from build123d import *

# Parameters (mm, degrees)
F0_W     = 127
F0_H     = 254
F1_DEPTH = 101.6
F3_DEPTH = 101.601


with BuildPart() as f1:
    # F0 (on Front) → F1 (new body)
    with BuildSketch(Plane.XZ):
        with Locations((-70.0115717482, 66.6608795685)):
            Rectangle(F0_W, F0_H)
    extrude(amount=F1_DEPTH)

    # F2 (on face) → F3 (cut, through all)
    with BuildSketch(Plane.XZ.offset(101.6)):
        with BuildLine():
            ThreePointArc((-133.5115717482, 89.8414792443), (-90.6735324782, 69.9836491161), (-61.4159074664, 107.0433631539))
            ThreePointArc((-61.4159074664, 107.0433631539), (-90.6735324782, 144.1030771918), (-133.5115717482, 124.2452470636))
            Line((-133.5115717482, 124.2452470636), (-133.5115717482, 89.8414792443))
        make_face()
    extrude(amount=-F3_DEPTH, mode=Mode.SUBTRACT)


solid = f1.part
Build history of the part. All positions in model axes, mm. Round coordinates to 2 decimals unless told otherwise and drop trailing zeros. Loops run counter-clockwise (first coordinate to the right, second up) from the corner with the lowest first, then second, coordinate; pieces in that order, holes last. Notation, with made-up numbers: (46, 45) -> (72, 45) arc R15 ccw to (72, 50) -> close; hole circle Ø3 at (46.5, -25). An arc over 180 degrees is marked (long way). Answer in a Markdown table with one row per item.
Item 1: Drill centre lines: L1, parallel to Z at x = -97.5, y = -71; L2, parallel to Z at x = -65.5, y = -63; L3, parallel to X at y = -79, z = 83. Where is each one in solid material? Low to high. Write a range as [from, to].
Answers below:
| item | result |
|---|---|
| L1 | z = [-60.34, 69], [145.09, 193.66] |
| L2 | z = [-60.34, 89.88], [124.21, 193.66] |
| L3 | x = [-133.51, -129.07], [-69.96, -6.51] |
Item 2: Saw through at C-C (z = 135). Write the cut outline in (x, y), and give its area (3 significant figures).
Answers below:
| item | result |
|---|---|
| outline | (-133.51, -101.6) -> (-125.4, -101.6) -> (-125.4, 0) -> (-133.51, 0) -> close; (-73.63, -101.6) -> (-6.51, -101.6) -> (-6.51, 0) -> (-73.63, 0) -> close |
| area | 7,640 mm² |
Item 3: Saw through at D-D (z = 99.5). Write the cut outline in (x, y), and give its area (3 significant figures).
Answers below:
| item | result |
|---|---|
| outline | (-62.17, -101.6) -> (-6.51, -101.6) -> (-6.51, 0) -> (-62.17, 0) -> close |
| area | 5,650 mm² |
Item 4: Saw through at A-A (x = -87). Write the cut outline in (y, z), and give its area (3 significant figures).
Answers below:
| item | result |
|---|---|
| outline | (-101.6, -60.34) -> (0, -60.34) -> (0, 71.06) -> (-101.6, 71.06) -> close; (-101.6, 143.03) -> (0, 143.03) -> (0, 193.66) -> (-101.6, 193.66) -> close |
| area | 18,500 mm² |
Item 5: Saw through at B-B (y = -48). Write the cut outline in (x, z), and give its area (3 significant figures).
Answers below:
| item | result |
|---|---|
| outline | (-133.51, -60.34) -> (-6.51, -60.34) -> (-6.51, 193.66) -> (-133.51, 193.66) -> (-133.51, 124.25) arc R38.1 cw (long way) to (-133.51, 89.84) -> close |
| area | 27,800 mm² |
